Autodesk Inventor part; units mm, degrees
ref_plane "Pracovní rovina2" through (10, 0, 0) normal (1, 0, 0) x (0, 0, -1)
ref_plane "YZ Plane" through (0, 0, 0) normal (1, 0, 0) x (0, 1, 0)
ref_plane "XZ Plane" through (0, 0, 0) normal (0, 1, 0) x (-1, 0, 0)
ref_plane "Pracovní rovina2" through (10, 0, 0) normal (1, 0, 0) x (0, 0, -1)
sketch "Náčrt1" plane through (10, 0, 0) normal (1, 0, 0) x (0, 0, -1)
  arc A0 (-3.3166, 5) -> (-3.3166, -5) centre (0, 0) ccw
  line L0 (3.3166, 5) -> (-3.3166, 5)
  arc A1 (3.3166, -5) -> (3.3166, 5) centre (0, 0) ccw
  line L1 (-3.3166, -5) -> (3.3166, -5)
  point P0 (0, 0)
extrude "Vysunutí1" add sketch "Náčrt1" along normal blind 15
sketch "Náčrt2" plane through (25, 0, 0) normal (1, 0, 0) x (0, 0, -1)
  line L0 (-6, 5) -> (-6, -5)
  line L1 (6, 5) -> (-6, 5)
  line L2 (6, 5) -> (6, -5)
  line L3 (-6, -5) -> (6, -5)
  point P0 (0, 0)
extrude "Vysunutí2" add sketch "Náčrt2" along normal blind 9
sketch "Náčrt3" plane through (34, 0, 0) normal (1, 0, 0) x (0, 0, -1)
  arc A0 (-1.3795, -0.589) -> (-0.4321, 1.4364) centre (0, 0) ccw
  line L0 (-1.3795, -0.589) -> (-0.4321, 1.4364)
  circle A1 centre (0, 0) radius 2
  arc A2 (-0.4321, 1.4364) -> (-1.3795, -0.589) centre (0, 0) ccw
extrude "Vysunutí3" add sketch "Náčrt3" along normal blind 1
extrude "Vysunutí4" add sketch "Náčrt3" along normal blind 10 contours L0 A0
extrude "Vysunutí5" add sketch "Náčrt3" along normal blind 1.8 contours A2 L0
sketch "Náčrt4" plane through (10, 0, 0) normal (-1, 0, 0) x (0, 0, 1)
  circle A0 centre (0, 0) radius 2.5
  dimension "d12" = 5
extrude "Vysunutí6" add sketch "Náčrt4" along normal blind 0.8
properties part number "GA12-N20 Motor_finalV"
Input: part model. Units: mm. Frame: model coordinates. A direction names the side the tool comes from. Give positions to 0.01 mm unless a question says otherwise; leave off trailing zeros. Order: outer loops, then holes, each group sorted by start corner. A loop starts at its lowest first (then second) coordinate and runs counter-clockwise, first axis right, second up. Notation, with made-up numbers: M 4.5,72.25 L 27.5,72.25 A25 cw 27.5,96.25 Z; hole C 42,35 d4. An arc over 180 degrees is marked long. One line per question, with ' | ' between items. Start each with the question number.
1. First-contact query: pin 1 Ø2 at (y, z) = (2, 5) entering from -X; pin 2 Ø1.5 at (x, z) = (20.5, -4.5) entering from -Y; pin 3 Ø1.5 at (x, z) = (38.5, 1.5) entering from +Y. Flat tips, straight axial feed; report the tip coordinate or a pass-through.
2. Section query A-A (z = 0). Return the cut outline in (x, y).
3. Section query C-C (x = 38.5). Return the cut outline in (y, z), and give its area (3 significant figures).
4. Access query for faces 5 (the face through (34, 2.3, 0.1)), 6 (the face through (17, 0, -6)), 7 (the face through (9.61, 2.44, -0.54)), 8 (the face through (17, 0, 6)), 9 (the face through (35.8, 0.5, 1.1)). Directions: +Z, -Z, +X, -X, +Y, -Y. A direction counts if a zero-diameter tool reaches every point of the face in a straight line with its end or side. Return the directions, or none.
5. Pull-direction query (Z, two-part tool) for faces 1 (the face through (39.843, 0.41, 0.912)), 2 (the face through (34.493, 1.952, 0.434)), 3 (the face through (29, 0, -6)), 4 (the face through (44, 0, 0)); classes: released by +Z, released by -Z, zero draft, split by the parting line, or undercut.
6. Section query B-B (y = 3.5). Return the cut outline in (x, z), and give its area (3 significant figures).
7. Material intervals for probe 1 along X at (y, z) = (4, 1); probe 2 along X at (y, z) = (-1.75, -1.5); probe 3 along Y at (x, z) = (21.5, 5.25), sorted ascending. Write a range as [from, to].
8. Section query D-D (z = -3). Return the cut outline in (x, y).
Here are the results:
1) pin 1: x = 10 | pin 2: y = -4.68 | pin 3: y = 0.76
2) outline: M 9.2,-2.5 L 10,-2.5 L 10,-5 L 34,-5 L 34,-2 L 35,-2 L 35,-1.5 L 44,-1.5 L 44,1.5 L 35,1.5 L 35,2 L 34,2 L 34,5 L 10,5 L 10,2.5 L 9.2,2.5 Z
3) outline: M -0.59,1.38 A1.5 ccw long 1.44,0.43 Z | area: 6.29 mm²
4) face 5: +X | face 6: -Z, -X | face 7: -X | face 8: +Z, -X | face 9: +Z, +X, +Y
5) face 1: released by +Z | face 2: split by the parting line | face 3: released by -Z | face 4: zero draft
6) outline: M 10,-4.87 L 25,-4.87 L 25,-6 L 34,-6 L 34,6 L 25,6 L 25,4.87 L 10,4.87 Z | area: 254 mm²
7) probe 1: [10, 34] | probe 2: [9.2, 34] | probe 3: [-2.9, 2.9]
8) outline: M 10,-5 L 34,-5 L 34,5 L 10,5 Z
